from build123d import *

# Parameters (mm, degrees)
SKIZZE1_R                       = 37.5
SKIZZE1_R_2                     = 3.25
AUFSATZ_LINEAR_AUSTRAGEN1_DEPTH = 9
BOHRUNG1_D                      = 6.7
BOHRUNG1_CBORE_D                = 11.1
BOHRUNG1_CBORE_DEPTH            = 5
SKIZZE3_R                       = 15.5
AUFSATZ_LINEAR_AUSTRAGEN2_DEPTH = 2
FASE1_SIZE                      = 0.5
SKIZZE7_R                       = 1.6
SCHNITT_LINEAR_AUSTRAGEN2_DEPTH = 55.161794653
FASE2_SIZE                      = 0.5
SKIZZE5_R                       = 2.9
AUFSATZ_LINEAR_AUSTRAGEN3_DEPTH = 3
FASE4_SIZE                      = 0.5


with BuildPart() as part:
    # Skizze1 → Aufsatz-Linear austragen1 (new body)
    with BuildSketch(Plane(origin=(0, 0, 0), x_dir=(1, 0, 0), z_dir=(0, 1, 0))):
        with Locations(Location((0, 0, 0), (0, 0, 270))):
            Circle(SKIZZE1_R)
        with Locations(Location((-25, 0, 0), (0, 0, 270))):
            Circle(SKIZZE1_R_2, mode=Mode.SUBTRACT)
        with Locations(Location((25, 0, 0), (0, 0, 270))):
            Circle(SKIZZE1_R_2, mode=Mode.SUBTRACT)
    extrude(amount=AUFSATZ_LINEAR_AUSTRAGEN1_DEPTH)

    # Bohrung1 (through all)
    with Locations(Plane(origin=(25, 0, 0), x_dir=(0, 0, -1), z_dir=(0, -1, 0))):
        with Locations((0, 0), (0, -50)):
            CounterBoreHole(BOHRUNG1_D / 2, BOHRUNG1_CBORE_D / 2, BOHRUNG1_CBORE_DEPTH)

    # Skizze3 → Aufsatz-Linear austragen2 (add)
    with BuildSketch(Plane(origin=(0, 9, 0), x_dir=(-1, 0, 0), z_dir=(0, 1, 0))):
        with Locations(Location((0, 0, 0), (0, 0, 90))):
            Circle(SKIZZE3_R)
    extrude(amount=AUFSATZ_LINEAR_AUSTRAGEN2_DEPTH)

    # Fase1
    fase1_edges = [part.edges().sort_by_distance(p)[0] for p in [
        (0, 11, -15.5),
    ]]
    chamfer(fase1_edges, length=FASE1_SIZE)

    # Skizze7 → Schnitt-Linear austragen2 (cut, through all)
    with BuildSketch(Plane(origin=(0, 0, 0), x_dir=(-1, 0, 0), z_dir=(0, -1, 0))):
        with Locations(Location((-15, 25, 0), (0, 0, 90))):
            Circle(SKIZZE7_R)
        with Locations(Location((15, 25, 0), (0, 0, 90))):
            Circle(SKIZZE7_R)
        with Locations(Location((15, -25, 0), (0, 0, 90))):
            Circle(SKIZZE7_R)
        with Locations(Location((-15, -25, 0), (0, 0, 90))):
            Circle(SKIZZE7_R)
    extrude(amount=-SCHNITT_LINEAR_AUSTRAGEN2_DEPTH, mode=Mode.SUBTRACT)

    # Fase2
    fase2_edges = [part.edges().sort_by_distance(p)[0] for p in [
        (0, 9, -37.5),
    ]]
    chamfer(fase2_edges, length=FASE2_SIZE)

    # Skizze5 → Aufsatz-Linear austragen3 (add)
    with BuildSketch(Plane(origin=(0, 9, 0), x_dir=(-1, 0, 0), z_dir=(0, 1, 0))):
        with Locations(Location((-17.67766953, 17.67766953, 0), (0, 0, 90))):
            Circle(SKIZZE5_R)
    extrude(amount=AUFSATZ_LINEAR_AUSTRAGEN3_DEPTH)

    # Fase4
    fase4_edges = [part.edges().sort_by_distance(p)[0] for p in [
        (17.67766953, 12, 14.77766953),
    ]]
    chamfer(fase4_edges, length=FASE4_SIZE)


solid = part.part
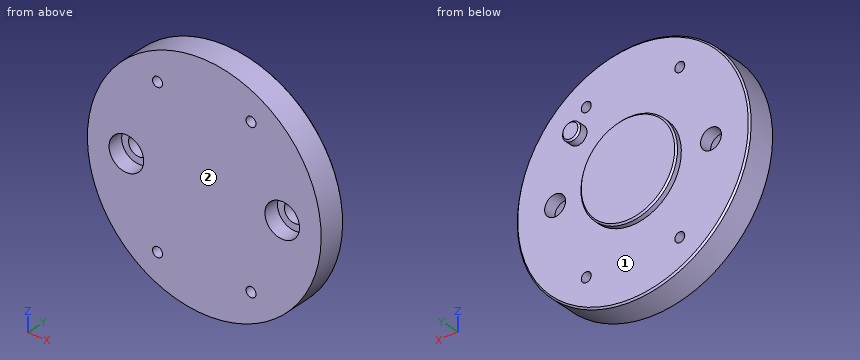
Work out the finished part from the listing and answer in its coordinate system (mm). Face numbers are marked on the shaded views. A direction names the side the tool comes from. Round coordinates to 2 decimals unless told otherwise and drop trailing zeros. Write each loop counter-clockwise with the first axis right and the second up, starting at its lowest first coordinate (ties: lowest second). Pieces come first, ordered by that corner, then holes. Notation, with made-up numbers: M -18.75,-7.75 L 39.25,-7.75 A9 ccw 39.25,-1.75 Z; hole C -23,75.25 d9. An arc over 180 degrees is marked long. Use a Markdown table: item, result.
1) The part is cut by section A-A on y = 3. Give the vertices of the cut face in (x, z), plus the area to 3 significant figures.
Taken from the geometry:
| item | result |
|---|---|
| outline | C 0,0 d75; hole C -25,0 d11.1; hole C -15,-25 d3.2; hole C -15,25 d3.2; hole C 15,-25 d3.2; hole C 15,25 d3.2; hole C 25,0 d11.1 |
| area | 4,190 mm2 |
2) The part is cut by section B-B on x = 0. Give the vertices of the cut face in (y, z), plus the area to 4 significant figures.
Taken from the geometry:
| item | result |
|---|---|
| outline | M 0,-37.5 L 8.5,-37.5 L 9,-37 L 9,-15.5 L 10.5,-15.5 L 11,-15 L 11,15 L 10.5,15.5 L 9,15.5 L 9,37 L 8.5,37.5 L 0,37.5 Z |
| area | 736.5 mm2 |
3) Consider line 1 (X direction, y = 2.5, z = -25); line 2 (X direction, y = 6.25, z = 0); line 3 (Y direction, x = -15, z = 28). Determine where each line is inside the solid, lowest interval first. Write a range as [from, to].
Taken from the geometry:
| item | result |
|---|---|
| line 1 | x = [-27.95, -16.6], [-13.4, 13.4], [16.6, 27.95] |
| line 2 | x = [-37.5, -28.35], [-21.65, 21.65], [28.35, 37.5] |
| line 3 | y = [0, 9] |
4) Flat-ended cylindrical pins translate along their axes: pin 1 (6 mm diameter, centred on y = 7.5, z = -27.5, fed in from -X); pin 2 (8.5 mm diameter, centred on x = 25, z = 0, fed in from -Y); pin 3 (2 mm diameter, centred on x = 4, y = 3.5, fed in from +Z); pin 4 (6 mm diameter, centred on x = 5.5, z = -25, fed in from -Y). Find the tip coordinate at first contact, or state that the pin passes through.
Taken from the geometry:
| item | result |
|---|---|
| pin 1 | stops at x = -28.39 |
| pin 2 | stops at y = 5 |
| pin 3 | stops at z = 37.38 |
| pin 4 | stops at y = 0 |
5) Which of the six approach directions +Z, -Z, +X, -X, +Y, -Y give full straight-line access (tool end or side, diameter ignored) to the marked faces 1 and 2?
Taken from the geometry:
| item | result |
|---|---|
| face 1 | +Y |
| face 2 | +Z, -Z, +X, -X, -Y |
6) The part is cut by section C-C on z = -25. State how many separate pieces and enclosed holes the cut face has, plus the area to 3 significant figures.
Taken from the geometry:
| item | result |
|---|---|
| separate pieces | 3 |
| enclosed holes | 0 |
| area | 445 mm2 |
